Check sheet for the modelled part. Datum: model origin and axes. Units: mm. Face numbers are marked on the shaded views. A direction names the side the tool comes from. Coordinates: 2 decimals unless noted, no trailing zeros. Loops run counter-clockwise (first coordinate to the right, second up) from the corner with the lowest first, then second, coordinate; pieces in that order, holes last.
```python
from build123d import *

# Parameters (mm, degrees)
BOSS_EXTRUDE1_DEPTH = 3


with BuildPart() as part:
    # Sketch1 → Boss-Extrude1 (new body)
    with BuildSketch(Plane(origin=(0, 0, 0), x_dir=(1, 0, 0), z_dir=(0, 1, 0))):
        with BuildLine():
            Line((-7.5, 2.5), (-10.5, 2.5))
            Line((-10.5, 2.5), (-10.5, -7.5))
            Line((-10.5, -7.5), (-7.5, -7.5))
            Line((-7.5, -7.5), (-2.5, -7.5))
            ThreePointArc((-2.5, -7.5), (4.571067812, -4.571067812), (7.5, 2.5))
            Line((7.5, 2.5), (7.5, 7.5))
            Line((7.5, 7.5), (7.5, 10.5))
            Line((7.5, 10.5), (-2.5, 10.5))
            Line((-2.5, 10.5), (-2.5, 7.5))
            Line((-2.5, 7.5), (-7.5, 7.5))
            Line((-7.5, 7.5), (-7.5, 2.5))
        make_face()
    extrude(amount=BOSS_EXTRUDE1_DEPTH)


solid = part.part
```
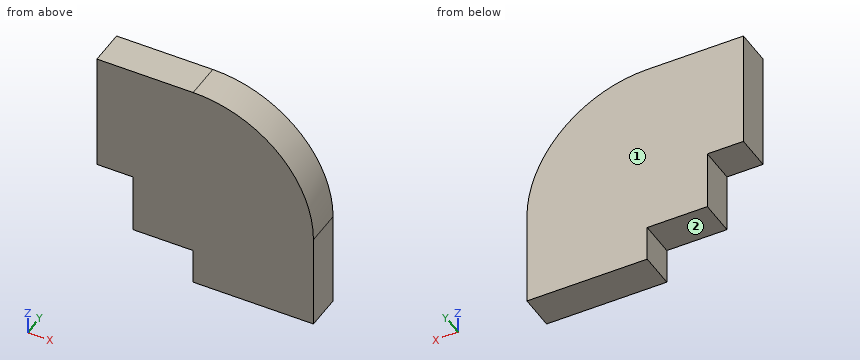
1) Section check B-B on z = -3. Enter the section's corners in (x, y).
Answer sheet:
outline: (-7.5, 0) - (7.5, 0) - (7.5, 3) - (-7.5, 3) - close
2) Section check A-A on y = 2. Enter the section's corners in (x, z).
Answer sheet:
outline: (-10.5, -2.5) - (-7.5, -2.5) - (-7.5, -7.5) - (-2.5, -7.5) - (-2.5, -10.5) - (7.5, -10.5) - (7.5, -2.5) arc R10 ccw to (-2.5, 7.5) - (-10.5, 7.5) - close
3) Section check C-C on x = -5.75. Enter the section's corners in (y, z).
Answer sheet:
outline: (0, -7.5) - (3, -7.5) - (3, 7.5) - (0, 7.5) - close
4) Depth check by flat-ended pin: pin 1 (0.9 mm diameter, centred on y = 1.5, z = -5.5, fed in from -X). Enter the tip coordinate at first touch or a pass-through.
Answer sheet:
pin 1: stops at x = -7.5
5) Scan lines: line 1 (X direction, y = 2.8, z = -5.25); line 2 (X direction, y = 2.35, z = -7.75). Record each from-to range of solid material in increasing order.
Answer sheet:
line 1: x = -7.5 to 7.5
line 2: x = -2.5 to 7.5
6) Set-up check for the marked faces 1 and 2: record each of +Z, -Z, +X, -X, +Y, -Y from which the full face is reachable in a straight line by a thin tool's end or side.
Answer sheet:
face 1: +Z, -Z, +X, -X, +Y
face 2: -Z, -X, +Y, -Y
